Part model, mm, in its own coordinate system. Face numbers are marked on the shaded views. Round coordinates to 2 decimals unless told otherwise and drop trailing zeros. Write each loop counter-clockwise with the first axis right and the second up, starting at its lowest first coordinate (ties: lowest second). Pieces come first, ordered by that corner, then holes. Notation, with made-up numbers: M 60.25,20.5 L 117.25,20.5 A21 ccw 117.25,34.5 Z; hole C 75.5,34 d4. An arc over 180 degrees is marked long. Answer as a JSON object with one key per item and string values. Group by question number.
1. Band-saw the part on A-A, the plane y = 5. Write the cut outline in (x, z), plus the area to 3 significant figures.
2. Band-saw the part on B-B, the plane y = -72.5. Write the cut outline in (x, z), plus the area to 3 significant figures.
3. Band-saw the part on D-D, the plane y = -153.5. Write the cut outline in (x, z), plus the area to 3 significant figures.
4. Band-saw the part on C-C, the plane z = 5.75. Count the separate pieces of the cut face and the enclosed holes in it, plus the area to 3 significant figures.
5. Two-plate mould, pull along X, no slides. Class the marked faces 1, 2 and 3: +X half, -X half, draft (parallel to the pull), parting line (faces both ways), or undercut.
6. Drop flat-ended pins along their axis: pin 1 (1.8 mm diameter, centred on x = 56.5, y = -80, fed in from +Z); pin 2 (2 mm diameter, centred on x = -0.5, z = 10, fed in from -Y); pin 3 (6 mm diameter, centred on x = -47, z = 3, fed in from +Y); pin 4 (8 mm diameter, centred on y = -106, z = 7, fed in from -X). Give the stop position or say it passes through.
7. Drill centre lines: line 1 (X direction, y = -115, z = 6.5); line 2 (Y direction, x = 1.5, z = 1.7); line 3 (X direction, y = -131, z = 11.5). Where is each one in solid material? Low to high. Write a range as from..to.
Autodesk Inventor part; units mm, degrees
ref_plane "YZ Plane" through (0, 0, 0) normal (1, 0, 0) x (0, 1, 0)
ref_plane "XZ Plane" through (0, 0, 0) normal (0, 1, 0) x (-1, 0, 0)
ref_plane "XY Plane" through (0, 0, 0) normal (0, 0, 1) x (1, 0, 0)
sketch "スケッチ1" plane through (0, 0, 0) normal (0, 0, 1) x (1, 0, 0)
  circle A0 centre (0, 0) radius 60
  circle A1 centre (0, 0) radius 7
  dimension "d0" = 120
  dimension "d1" = 14
extrude "押し出し1" add sketch "スケッチ1" along normal blind 3
sketch "スケッチ2" plane through (0, 0, 3) normal (0, 0, 1) x (1, 0, 0)
  circle A0 centre (0, 0) radius 46
  line L0 (0, 0) -> (0, 59.211)
  line L1 (0, 0) -> (-21.8609, 52.777)
  line L2 (0, 0) -> (27.8226, 47.8581)
  point P0 (-17.6034, 42.4985)
  point P1 (-42.4985, 17.6034)
  point P2 (-42.4985, -17.6034)
  point P3 (-17.6034, -42.4985)
  point P4 (17.6034, -42.4985)
  point P5 (42.4985, -17.6034)
  point P6 (42.4985, 17.6034)
  point P7 (17.6034, 42.4985)
  dimension "d4" = 92
  dimension "d5" = 22.5
  dimension "d8" = 360
hole "穴1" at (-17.6034, 42.4985, 3) at (-42.4985, 17.6034, 3) at (-42.4985, -17.6034, 3) at (-17.6034, -42.4985, 3) at (17.6034, -42.4985, 3) at (42.4985, -17.6034, 3) at (42.4985, 17.6034, 3) at (17.6034, 42.4985, 3) direction (0, 0, -1) diameter 3 end through all
sketch "スケッチ4" plane through (0, 0, 0) normal (0, 0, -1) x (-1, 0, 0)
  line L0 (0, 0) -> (0, -80.557)
  circle A0 centre (0, 0) radius 60
  line L1 (-60, 0) -> (-60, -210)
  line L2 (60, 0) -> (60, -210)
  line L3 (-60, -210) -> (60, -210)
  line L4 (-60, 0) -> (-41.6274, -210)
  line L5 (60, 0) -> (41.6274, -210)
  line L6 (12.7278, -162.7278) -> (60, -210)
  line L7 (19.706, -169.706) -> (-7.6224, -142.3776)
  line L8 (0, -80.557) -> (0, -150)
  line L9 (7, -239.3448) -> (7, -80.557)
  line L10 (7, -80.557) -> (7, 0)
  line L11 (7, -239.3448) -> (7, -157)
  circle A1 centre (0, 0) radius 7
  point P0 (60, 0)
  point P1 (60, 0)
  point P2 (-59.0885, -10.4189)
  point P3 (-58.5, -13.3323)
  point P4 (57, -18.735)
  point P5 (59.0885, -10.4189)
  point P6 (7, -136.3384)
  point P7 (7, -59.5903)
  point P8 (43.1055, -193.1055)
  point P9 (7, -210)
  point P10 (7, -136.3384)
  point P11 (7, -157)
  dimension "d21" = 60
  dimension "d23" = 120
  dimension "d24" = 210
  dimension "d25" = 210
  dimension "d56" = 0
  dimension "d89" = 85
  dimension "d90" = 85
  dimension "d207" = 45
  dimension "d208" = 7
extrude "押し出し3" add sketch "スケッチ4" against normal blind 3 contours A0 L10 L9 L7 L8 L0 | L0 L8 L7 L9 L3 L4 A0 | L4 L3 L1 A0 | L7 L6 L5 L3 L9 | L6 L3 L5
sketch "スケッチ17" plane through (0, 0, 3) normal (0, 0, 1) x (1, 0, 0)
  circle A0 centre (0, 0) radius 30
  dimension "d159" = 60
extrude "押し出し10" cut sketch "スケッチ17" against normal blind 10
sketch "スケッチ20" plane through (0, 0, 3) normal (0, 0, 1) x (1, 0, 0)
  line L0 (-60, -210) -> (60, -210)
  circle A0 centre (0, 0) radius 30
  line L1 (60, -210) -> (60, 0)
  point P0 (1.5, -179.9937)
  point P1 (0, -210)
  point P2 (58.5, -136.6677)
  point P3 (51.5, -210)
  point P4 (48.5, -124.0626)
  point P5 (60, -150)
  dimension "d205" = 180
  dimension "d223" = 58.5
  dimension "d246" = 60
hole "穴8" at (1.5, -179.9937, 3) direction (0, 0, -1) diameter 10 end through all
fillet "フィレット4" radius 10 2 edges at (-60, -210, 1.5) (60, -210, 1.5)
fillet "フィレット5" radius 10 2 edges at (-7, -59.5903, 1.5) (60, 0, 1.5)
sketch "スケッチ23" plane through (0, 0, 3) normal (0, 0, 1) x (1, 0, 0)
  circle A0 centre (0, 0) radius 60
  circle A1 centre (0, 0) radius 53
  arc A2 (-7, -67.9043) -> (-14.5714, -58.2037) centre (-17, -67.9043) ccw
  line L0 (-7, -67.9043) -> (-7, -157)
  line L1 (60, -157) -> (60, 0)
  line L2 (0, -157) -> (0, -60)
  line L3 (-7, -67.9043) -> (-7, -59.5903)
  line L4 (53, 0) -> (53, -150)
  line L5 (53, -150) -> (0, -150)
  line L6 (0, -150) -> (0, -67.9043)
  line L7 (0, -67.9043) -> (0, -59.5903)
  line L8 (53, -150) -> (53, -157)
  line L9 (0, -59.5903) -> (0, -53)
  line L10 (-35.8579, -210) -> (50, -210)
  line L11 (-7, -150) -> (60, -150)
  point P0 (-7, -112.4522)
  point P1 (53, 0)
  point P2 (53, -28.1247)
  dimension "d247" = 120
  dimension "d248" = 7
  dimension "d249" = 7
  dimension "d250" = 7
  dimension "d267" = 60
extrude "押し出し14" add sketch "スケッチ23" along normal blind 12.3 contours A0 L4 A1 L9 L7 | L1 L11 L4 A0 | A0 L3 A2 | A0 L2 L11 L0 L3 picked at (54.2848, -15.7658)
sketch "スケッチ24" plane through (0, 0, 15.3) normal (0, 0, 1) x (1, 0, 0)
  circle A0 centre (0, 0) radius 60
  circle A1 centre (0, 0) radius 56.5
  circle A2 centre (-17.6034, 42.4985) radius 1.5
  line L0 (0, 0) -> (-17.6034, 42.4985)
  line L1 (-17.6034, 42.4985) -> (-25.261, 60.9855)
  point P0 (-21.6216, 52.1992)
  point P1 (-52.1992, 21.6216)
  point P2 (-52.1992, -21.6216)
  point P3 (-21.6216, -52.1992)
  point P4 (21.6216, -52.1992)
  point P5 (52.1992, -21.6216)
  point P6 (52.1992, 21.6216)
  point P7 (21.6216, 52.1992)
  dimension "d253" = 120
  dimension "d254" = 3.5
  dimension "d257" = 360
hole "穴10" at (-21.6216, -52.1992, 15.3) at (-52.1992, -21.6216, 15.3) at (-52.1992, 21.6216, 15.3) at (-21.6216, 52.1992, 15.3) at (21.6216, 52.1992, 15.3) at (52.1992, 21.6216, 15.3) direction (0, 0, -1) diameter 3 end through all
sketch "スケッチ25" plane through (0, 0, 15.3) normal (0, 0, 1) x (1, 0, 0)
  line L0 (-7, -150) -> (0, -150)
  line L1 (-7, -67.9043) -> (-7, -150)
  line L2 (60, -150) -> (60, 0)
  line L3 (53, -150) -> (60, -150)
  point P0 (0, 0)
  point P1 (-3.5, -80)
  point P2 (56.5, -80)
  point P3 (-3.5, -115)
  point P4 (56.5, -115)
  point P5 (56.5, -45)
  point P6 (56.5, -10)
  point P7 (-3.5, -150)
  point P8 (56.5, -150)
  dimension "d268" = 35
  dimension "d269" = 35
  dimension "d270" = 3.5
  dimension "d271" = 3.5
  dimension "d272" = 3.5
  dimension "d273" = 3.5
  dimension "d274" = 3.5
  dimension "d275" = 3.5
  dimension "d276" = 35
  dimension "d277" = 35
  dimension "d278" = 35
  dimension "d279" = 35
hole "穴11" at (-3.5, -80, 15.3) at (56.5, -80, 15.3) at (-3.5, -115, 15.3) at (56.5, -115, 15.3) at (56.5, -45, 15.3) at (56.5, -10, 15.3) direction (0, 0, -1) diameter 3 end through all
fillet "フィレット8" radius 3.5 4 edges at (-7, -150, 9.15) (0, -150, 9.15) (53, -150, 9.15) (60, -150, 9.15)
fillet "フィレット9" radius 10 1 edges at (0, -53, 9.15)
equation "\"d25\" = d24"
equation "\"d90\" = d89"
properties part number "legparts_08(seven)" material "ABS プラスチック"
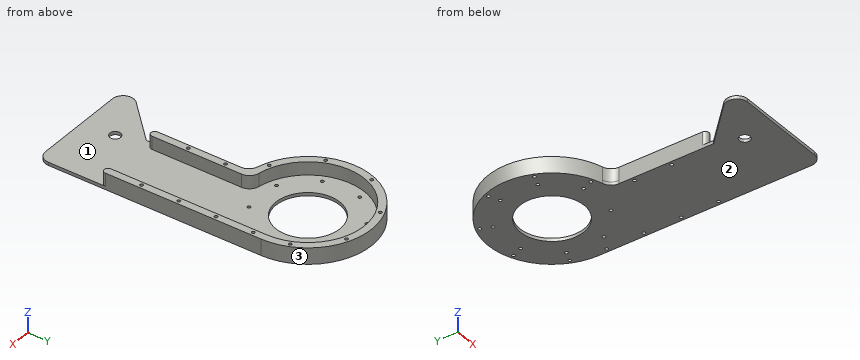
Worked answers:
{
 "1": {"outline": "M -59.79,0 L -29.58,0 L -29.58,3 L -52.76,3 L -52.76,15.3 L -59.79,15.3 Z; M 29.58,0 L 59.79,0 L 59.79,15.3 L 52.76,15.3 L 52.76,3 L 29.58,3 Z", "area": "354 mm^2"},
 "2": {"outline": "M -7,0 L 60,0 L 60,15.3 L 53,15.3 L 53,3 L 0,3 L 0,15.3 L -7,15.3 Z", "area": "373 mm^2"},
 "3": {"outline": "M -7,0 L 60,0 L 60,3 L -7,3 Z", "area": "201 mm^2"},
 "4": {"separate pieces": "1", "enclosed holes": "12", "area": "3,450 mm^2"},
 "5": {"face 1": "undercut", "face 2": "draft", "face 3": "parting line"},
 "6": {"pin 1": "passes through", "pin 2": "stops at y = -149.37", "pin 3": "stops at y = 40.79", "pin 4": "stops at x = -7"},
 "7": {"line 1": "x = -7..-5, -2..0, 53..55, 58..60", "line 2": "y = -210..-184.99, -174.99..-29.96, 29.96..59.98", "line 3": "x = -7..0, 53..60"}
}
